Source: CAD feature listing. Evaluate the final solid. Frame: model axes, mm. A direction names the side the tool comes from. Give positions to 0.01 mm unless a question says otherwise; leave off trailing zeros. Loops run counter-clockwise (first coordinate to the right, second up) from the corner with the lowest first, then second, coordinate; pieces in that order, holes last. Notation, with made-up numbers: M -33,63.5 L 25,63.5 A25 cw 25,82.5 Z; hole C -38.75,40 d9. An arc over 180 degrees is marked long. Answer in a Markdown table with one row per item.
```python
from build123d import *

# Parameters (mm, degrees)
ESQUISSE1_W             = 27.85
ESQUISSE1_H             = 200
BOSS_EXTRU_1_DEPTH      = 6
ESQUISSE4_W             = 7.790942256
ESQUISSE4_H             = 7.790942256
ESQUISSE4_R             = 3
ENL_V_MAT_EXTRU_3_DEPTH = 29
ESQUISSE5_R             = 13.925
ENL_V_MAT_EXTRU_4_DEPTH = 3
ESQUISSE7_W             = 16.87
ESQUISSE7_H             = 23
ESQUISSE7_H_2           = 29
ENL_V_MAT_EXTRU_6_DEPTH = 13
CONG_1_R                = 10
CONG_2_R                = 10
ESQUISSE8_R             = 1.6
ENL_V_MAT_EXTRU_7_DEPTH = 10
ESQUISSE11_W            = 20.3
ESQUISSE11_H            = 40.6
ENL_V_MAT_EXTRU_8_DEPTH = 1.85
ESQUISSE12_W            = 27.85
ESQUISSE12_H            = 6.85
BOSS_EXTRU_5_DEPTH      = 31.25
ESQUISSE14_W            = 10
ESQUISSE14_H            = 20
ESQUISSE14_H_2          = 3
BOSS_EXTRU_6_DEPTH      = 1
ESQUISSE15_W            = 3
ESQUISSE15_H            = 30.75
BOSS_EXTRU_7_DEPTH      = 31.25
TROU_TARAUD_M32_D       = 2.5
TROU_TARAUD_M32_DEPTH   = 8.5
TROU_TARAUD_M32_TIP     = 0.751075774


with BuildPart() as part:
    # Esquisse1 → Boss.-Extru.1 (new body)
    with BuildSketch(Plane.XY):
        with Locations((4.111190476, -68.237738095)):
            Rectangle(ESQUISSE1_W, ESQUISSE1_H)
        with BuildLine():
            Line((-9.813809524, 31.762261905), (18.036190476, 31.762261905))
            ThreePointArc((18.036190476, 31.762261905), (4.111190476, 45.687261905), (-9.813809524, 31.762261905))
        make_face()
    extrude(amount=BOSS_EXTRU_1_DEPTH)

    # Esquisse4 → Enlèv. mat.-Extru.3 (cut)
    # profile 1 of 9: a face of its own
    with BuildSketch(Plane.XY.offset(6)):
        Polygon((4.111190476, -154.728709994), (2.615719348, -156.342266967), (5.606661604, -156.342266967), align=None)
    # profile 2 of 9: a face of its own
    with BuildSketch(Plane.XY.offset(6)):
        with Locations((4.111190476, -160.237738095)):
            Rectangle(ESQUISSE4_W, ESQUISSE4_H)
        with Locations((4.111190476, -160.237738095)):
            Circle(ESQUISSE4_R, mode=Mode.SUBTRACT)
    # profile 3 of 9: a face of its own
    with BuildSketch(Plane.XY.offset(6)):
        Polygon((0.215719348, -161.733209223), (0.215719348, -158.742266967), (-1.397837625, -160.237738095), align=None)
    # profile 4 of 9: a face of its own
    with BuildSketch(Plane.XY.offset(6)):
        Polygon((5.606661604, -164.133209223), (2.615719348, -164.133209223), (4.111190476, -165.746766196), align=None)
    # profile 5 of 9: a face of its own
    with BuildSketch(Plane.XY.offset(6)):
        Polygon((9.620218577, -160.237738095), (8.006661604, -158.742266967), (8.006661604, -161.733209223), align=None)
    # profile 6 of 9: a face of its own
    with BuildSketch(Plane.XY.offset(6)):
        with BuildLine():
            ThreePointArc((7.111190476, -160.237738095), (4.887647611, -157.339960616), (1.513114265, -158.737738095))
            Line((1.513114265, -158.737738095), (1.513114265, -161.737738095))
            ThreePointArc((1.513114265, -161.737738095), (4.887647611, -163.135515574), (7.111190476, -160.237738095))
        make_face()
    # profile 7 of 9: a face of its own
    with BuildSketch(Plane.XY.offset(6)):
        with BuildLine():
            Line((1.513114265, -161.737738095), (1.513114265, -158.737738095))
            ThreePointArc((1.513114265, -158.737738095), (1.111190476, -160.237738095), (1.513114265, -161.737738095))
        make_face()
    # profile 8 of 9: a face of its own
    with BuildSketch(Plane.XY.offset(6)):
        with BuildLine():
            ThreePointArc((7.111190476, -160.237738095), (4.887647611, -157.339960616), (1.513114265, -158.737738095))
            Line((1.513114265, -158.737738095), (1.513114265, -161.737738095))
            ThreePointArc((1.513114265, -161.737738095), (4.887647611, -163.135515574), (7.111190476, -160.237738095))
        make_face()
    # profile 9 of 9: a face of its own
    with BuildSketch(Plane.XY.offset(6)):
        with BuildLine():
            Line((1.513114265, -161.737738095), (1.513114265, -158.737738095))
            ThreePointArc((1.513114265, -158.737738095), (1.111190476, -160.237738095), (1.513114265, -161.737738095))
        make_face()
    extrude(amount=-ENL_V_MAT_EXTRU_3_DEPTH, mode=Mode.SUBTRACT)

    # Esquisse5 → Enlèv. mat.-Extru.4 (cut)
    with BuildSketch(Plane(origin=(0, 0, 0), x_dir=(-1, 0, 0), z_dir=(0, 0, -1))):
        with Locations((-4.111190476, 31.762261905)):
            Circle(ESQUISSE5_R)
    extrude(amount=-ENL_V_MAT_EXTRU_4_DEPTH, mode=Mode.SUBTRACT)

    # Esquisse7 → Enlèv. mat.-Extru.6 (cut)
    with BuildSketch(Plane(origin=(0, 0, 0), x_dir=(-1, 0, 0), z_dir=(0, 0, -1))):
        with BuildLine():
            ThreePointArc((-13.036190476, -115.237738095), (-4.601190476, -106.802738095), (3.833809524, -115.237738095))
            Line((3.833809524, -115.237738095), (-13.036190476, -115.237738095))
        make_face()
        with Locations((-4.601190476, -126.737738095)):
            Rectangle(ESQUISSE7_W, ESQUISSE7_H)
        with BuildLine():
            Line((-13.036190476, -138.237738095), (3.833809524, -138.237738095))
            ThreePointArc((3.833809524, -138.237738095), (-4.601190476, -146.672738095), (-13.036190476, -138.237738095))
        make_face()
        with BuildLine():
            Line((3.833809524, -93.237738095), (-13.036190476, -93.237738095))
            ThreePointArc((-13.036190476, -93.237738095), (-4.601190476, -101.672738095), (3.833809524, -93.237738095))
        make_face()
        with Locations((-4.601190476, -78.737738095)):
            Rectangle(ESQUISSE7_W, ESQUISSE7_H_2)
        with BuildLine():
            Line((3.833809524, -64.237738095), (-13.036190476, -64.237738095))
            ThreePointArc((-13.036190476, -64.237738095), (-4.601190476, -55.802738095), (3.833809524, -64.237738095))
        make_face()
        with BuildLine():
            ThreePointArc((3.833809524, -42.237738095), (-4.601190476, -50.672738095), (-13.036190476, -42.237738095))
            Line((-13.036190476, -42.237738095), (3.833809524, -42.237738095))
        make_face()
        with Locations((-4.601190476, -30.737738095)):
            Rectangle(ESQUISSE7_W, ESQUISSE7_H)
        with BuildLine():
            Line((3.833809524, -19.237738095), (-13.036190476, -19.237738095))
            ThreePointArc((-13.036190476, -19.237738095), (-4.601190476, -10.802738095), (3.833809524, -19.237738095))
        make_face()
    extrude(amount=-ENL_V_MAT_EXTRU_6_DEPTH, mode=Mode.SUBTRACT)

    # Congé1
    cong_1_edges = [part.edges().sort_by_distance(p)[0] for p in [
        (18.036190476, -168.237738095, 3),
    ]]
    fillet(cong_1_edges, radius=CONG_1_R)

    # Congé2
    cong_2_edges = [part.edges().sort_by_distance(p)[0] for p in [
        (-9.813809524, -168.237738095, 3),
    ]]
    fillet(cong_2_edges, radius=CONG_2_R)

    # Esquisse8 → Enlèv. mat.-Extru.7 (cut)
    with BuildSketch(Plane(origin=(0, 0, 3), x_dir=(-1, 0, 0), z_dir=(0, 0, -1))):
        with Locations((-4.111190476, 31.762261905)):
            Circle(ESQUISSE8_R)
    extrude(amount=-ENL_V_MAT_EXTRU_7_DEPTH, mode=Mode.SUBTRACT)

    # Esquisse11 → Enlèv. mat.-Extru.8 (cut)
    with BuildSketch(Plane.XY.offset(6)):
        with Locations((4.111190476, 21.312261905)):
            Rectangle(ESQUISSE11_W, ESQUISSE11_H)
    extrude(amount=-ENL_V_MAT_EXTRU_8_DEPTH, mode=Mode.SUBTRACT)

    # Esquisse12 → Boss.-Extru.5 (add)
    with BuildSketch(Plane.XY.offset(6)):
        with Locations((4.111190476, -2.412738095)):
            Rectangle(ESQUISSE12_W, ESQUISSE12_H)
    extrude(amount=BOSS_EXTRU_5_DEPTH)

    # Esquisse14 → Boss.-Extru.6 (add)
    with BuildSketch(Plane.XY.offset(4.15)):
        with Locations((4.111190476, 11.012261905)):
            Rectangle(ESQUISSE14_W, ESQUISSE14_H)
        with Locations((4.111190476, 40.112261905)):
            Rectangle(ESQUISSE14_W, ESQUISSE14_H_2)
    extrude(amount=BOSS_EXTRU_6_DEPTH)

    # Esquisse15 → Boss.-Extru.7 (add)
    with BuildSketch(Plane.XY.offset(6)):
        with Locations((-8.313809524, 16.387261905)):
            Rectangle(ESQUISSE15_W, ESQUISSE15_H)
        with Locations((16.536190476, 16.387261905)):
            Rectangle(ESQUISSE15_W, ESQUISSE15_H)
    extrude(amount=BOSS_EXTRU_7_DEPTH)

    # Trou taraudé M32
    with Locations(Plane.XY.offset(37.25)):
        with Locations((-0.893809524, -2.807738095), (9.106190476, -2.807738095)):
            Hole(TROU_TARAUD_M32_D / 2, depth=TROU_TARAUD_M32_DEPTH)
            with Locations((0, 0, -(TROU_TARAUD_M32_DEPTH + TROU_TARAUD_M32_TIP / 2))):  # 118° drill point
                Cone(0, TROU_TARAUD_M32_D / 2, TROU_TARAUD_M32_TIP, mode=Mode.SUBTRACT)


solid = part.part
```
Q1. Ray query, probe 1 along Y at (x, z) = (-8.5, 25); probe 2 along X at (y, z) = (-115, 5); probe 3 along Y at (x, z) = (13, 32). Return the intervals inside material, ascending. Write a range as from..to.
Values follow:
| item | result |
|---|---|
| probe 1 | -5.84..31.76 |
| probe 2 | -9.81..-3.83, 13.03..18.04 |
| probe 3 | -5.84..1.01 |
Q2. Section query D-D (y = 23.5). Output: boundary loops of the cut face in (x, z), plus the area to 3 significant figures.
Values follow:
| item | result |
|---|---|
| outline | M -9.81,0 L -7.1,0 L -7.1,3 L 15.32,3 L 15.32,0 L 18.04,0 L 18.04,37.25 L 15.04,37.25 L 15.04,6 L 14.26,6 L 14.26,4.15 L -6.04,4.15 L -6.04,6 L -6.81,6 L -6.81,37.25 L -9.81,37.25 Z |
| area | 250 mm^2 |
Q3. Section query C-C (y = -95). Output: boundary loops of the cut face in (x, z), plus the area to 3 significant figures.
Values follow:
| item | result |
|---|---|
| outline | M -9.81,0 L -3.65,0 L -3.65,6 L -9.81,6 Z; M 12.85,0 L 18.04,0 L 18.04,6 L 12.85,6 Z |
| area | 68.1 mm^2 |
Q4. Reachability of faces 1 (the cylindrical face through (4.42, -146.67, 2.96)), 2 (the flat face through (4, 11, 5.15)), 3 (the flat face through (4, -5.838, 21)) from +Z, -Z, +X, -X, +Y, -Y: full face, straight path, thin tool, end or side. Return the list, or none.
Values follow:
| item | result |
|---|---|
| face 1 | +Z, -Z |
| face 2 | +Z |
| face 3 | +Z, +X, -X, -Y |
Q5. Contact query for flat-ended pins moving along their axis: pin 1 Ø1.5 at (x, z) = (-8, 29.5) entering from +Y; pin 2 Ø6 at (x, y) = (15, -103) entering from +Z; pin 3 Ø5 at (x, z) = (0, 32) entering from +Y. Output: stop coordinate, or through.
Values follow:
| item | result |
|---|---|
| pin 1 | y = 31.76 |
| pin 2 | z = 6 |
| pin 3 | y = 1.01 |
Q6. Section query A-A (y = -70.5). Output: boundary loops of the cut face in (x, z), plus the area to 3 significant figures.
Values follow:
| item | result |
|---|---|
| outline | M -9.81,0 L -3.83,0 L -3.83,6 L -9.81,6 Z; M 13.04,0 L 18.04,0 L 18.04,6 L 13.04,6 Z |
| area | 65.9 mm^2 |
Q7. Mould query, pull axis Y, two halves, no side actions, for faces 4 (the flat face through (15.036, 16, 21)), 5 (the cylindrical face through (4.417, 45.684, 4.479)), 6 (the flat face through (-3.834, -79, 3)). Classes: +Y half, -Y half, draft (parallel to the pull), parting line (faces both ways), or undercut.
Values follow:
| item | result |
|---|---|
| face 4 | draft |
| face 5 | +Y half |
| face 6 | undercut |
Q8. Section query B-B (z = 17). Output: boundary loops of the cut face in (x, y), plus the area to 3 significant figures.
Values follow:
| item | result |
|---|---|
| outline | M -9.81,-5.84 L 18.04,-5.84 L 18.04,31.76 L 15.04,31.76 L 15.04,1.01 L -6.81,1.01 L -6.81,31.76 L -9.81,31.76 Z |
| area | 375 mm^2 |
